from build123d import *

# Parameters (mm, degrees)
ESBO_O1_W                = 7
ESBO_O1_H                = 3
ESBO_O1_W_2              = 53
ESBO_O1_H_2              = 27
ESBO_O1_H_3              = 7
ESBO_O1_R                = 1.55
RESSALTO_EXTRUS_O1_DEPTH = 2
ESBO_O2_W                = 7
ESBO_O2_H                = 3
RESSALTO_EXTRUS_O2_DEPTH = 14
ESBO_O3_W                = 7
ESBO_O3_H                = 2
RESSALTO_EXTRUS_O3_DEPTH = 2
FILETE1_R                = 2
FILETE2_R                = 3
ESBO_O4_R                = 1.55
CORTE_EXTRUS_O1_DEPTH    = 2
FILETE3_R                = 2


with BuildPart() as part:
    # Esboço1 → Ressalto-extrusão1 (new body)
    # profile 1 of 3: a face of its own
    with BuildSketch(Plane(origin=(0, 0, 0), x_dir=(1, 0, 0), z_dir=(0, 1, 0))):
        with Locations((-23, -15)):
            Rectangle(ESBO_O1_W, ESBO_O1_H)
    # profile 2 of 3: a face of its own
    with BuildSketch(Plane(origin=(0, 0, 0), x_dir=(1, 0, 0), z_dir=(0, 1, 0))):
        Rectangle(ESBO_O1_W_2, ESBO_O1_H_2)
    # profile 3 of 3: a face of its own
    with BuildSketch(Plane(origin=(0, 0, 0), x_dir=(1, 0, 0), z_dir=(0, 1, 0))):
        with Locations((-23, 17)):
            Rectangle(ESBO_O1_W, ESBO_O1_H_3)
        with Locations(Location((-23, 17, 0), (0, 0, 270))):
            Circle(ESBO_O1_R, mode=Mode.SUBTRACT)
    extrude(amount=-RESSALTO_EXTRUS_O1_DEPTH)

    # Esboço2 → Ressalto-extrusão2 (add)
    with BuildSketch(Plane(origin=(0, 0, 0), x_dir=(1, 0, 0), z_dir=(0, 1, 0))):
        with Locations((-23, -15)):
            Rectangle(ESBO_O2_W, ESBO_O2_H)
    extrude(amount=RESSALTO_EXTRUS_O2_DEPTH)

    # Esboço3 → Ressalto-extrusão3 (add)
    with BuildSketch(Plane(origin=(0, 0, 13.5), x_dir=(-1, 0, 0), z_dir=(0, 0, -1))):
        with Locations((23, 13)):
            Rectangle(ESBO_O3_W, ESBO_O3_H)
    extrude(amount=RESSALTO_EXTRUS_O3_DEPTH)

    # Filete1
    filete1_edges = [part.edges().sort_by_distance(p)[0] for p in [
        (-23, 12, 13.5),
    ]]
    fillet(filete1_edges, radius=FILETE1_R - 0.0001)  # a hair under: the kernel refuses the full size

    # Filete2
    filete2_edges = [part.edges().sort_by_distance(p)[0] for p in [
        (-19.5, -1, 13.5),
    ]]
    fillet(filete2_edges, radius=FILETE2_R - 0.0001)  # a hair under: the kernel refuses the full size

    # Esboço4 → Corte-extrusão1 (cut)
    with BuildSketch(Plane(origin=(0, 0, 0), x_dir=(1, 0, 0), z_dir=(0, 1, 0))):
        with Locations(Location((22.5, 0, 0), (0, 0, 270))):
            Circle(ESBO_O4_R)
    extrude(amount=-CORTE_EXTRUS_O1_DEPTH, mode=Mode.SUBTRACT)

    # Filete3
    filete3_edges = [part.edges().sort_by_distance(p)[0] for p in [
        (-26.5, -1, -20.5),
        (-19.5, -1, -20.5),
        (26.5, -1, -13.5),
        (26.5, -1, 13.5),
    ]]
    fillet(filete3_edges, radius=FILETE3_R)


solid = part.part
Source: CAD feature listing. Evaluate the final solid. Frame: model axes, mm. A direction names the side the tool comes from. Round coordinates to 2 decimals unless told otherwise and drop trailing zeros. Loops run counter-clockwise (first coordinate to the right, second up) from the corner with the lowest first, then second, coordinate; pieces in that order, holes last. Notation, with made-up numbers: (83, 15.5) - (140, 15.5) arc R14 cw to (140, 34.5) - close; hole circle Ø5 at (76.5, 80). An arc over 180 degrees is marked (long way). Write item = value, one per line. Start each with the question number.
Item 1: Reachability of faces 5 (the face through (4, -1, 13.5)), 6 (the face through (-23.05, 11.4, 12.93)), 7 (the face through (-19.5, -1, -16)) from +Z, -Z, +X, -X, +Y, -Y: full face, straight path, thin tool, end or side. Return the list, or none.
Item 2: Section query B-B on z = 0. Output: boundary loops of the cut face in (x, y).
Item 3: Mould query, pull axis X, two halves, no side actions, for faces 1 (the face through (-19.5, 8, 15)), 2 (the face through (-21.463, -0.986, -17.202)), 3 (the face through (-25.93, -1.01, -19.9)), 4 (the face through (24.037, -0.986, -0.202)). Classes: released by +X, released by -X, zero draft, split by the parting line, or undercut.
Item 4: First-contact query: pin 1 Ø1.6 at (x, y) = (0, -1.5) entering from +Z; pin 2 Ø1.6 at (x, y) = (-5, -1) entering from -Z; pin 3 Ø3.5 at (x, y) = (-24, 4.5) entering from -Z; pin 4 Ø3 at (x, z) = (22.5, 0) entering from -Y. Flat tips, straight axial feed; report the tip coordinate or a pass-through.
Item 5: Section query A-A on x = 22.5. Output: boundary loops of the cut face in (y, z).
Item 6: Section query D-D on x = 9.5. Output: boundary loops of the cut face in (y, z), plus the area to 3 significant figures.
Item 7: Material intervals for line 1 (X direction, y = -0.8, z = 0); line 2 (X direction, y = -0.8, z = -17); line 3 (Y direction, x = -8, z = 11), sorted ascending.
Results list:
q1.face_5 = +Z, +X, +Y, -Y
q1.face_6 = -Z, +X, -X
q1.face_7 = -Z, +X, +Y, -Y
q2.outline = (-26.5, -2) - (20.95, -2) - (20.95, 0) - (-26.5, 0) - close; (24.05, -2) - (26.5, -2) - (26.5, 0) - (24.05, 0) - close
q3.face_1 = released by +X
q3.face_2 = undercut
q3.face_3 = released by -X
q3.face_4 = undercut
q4.pin_1 = 13.5
q4.pin_2 = -13.5
q4.pin_3 = 13.5
q4.pin_4 = through
q5.outline = (-2, -13.5) - (0, -13.5) - (0, -1.55) - (-2, -1.55) - close; (-2, 1.55) - (0, 1.55) - (0, 13.5) - (-2, 13.5) - close
q6.outline = (-2, -13.5) - (0, -13.5) - (0, 13.5) - (-2, 13.5) - close
q6.area = 54.0 mm²
q7.line_1 = -26.5 to 20.95, 24.05 to 26.5
q7.line_2 = -26.5 to -24.55, -21.45 to -19.5
q7.line_3 = -2 to 0
